Here's how the part is built. I have some questions about the finished solid (model axes, mm). A direction names the side the tool comes from. Give positions to 0.01 mm unless a question says otherwise; leave off trailing zeros. Loops run counter-clockwise (first coordinate to the right, second up) from the corner with the lowest first, then second, coordinate; pieces in that order, holes last. Notation, with made-up numbers: (15, -12.5) - (27, -12.5) arc R17 cw to (27, -6.5) - close; hole circle Ø5 at (-0.5, 2.25). An arc over 180 degrees is marked (long way). Return JSON: item names as keys, results as strings. Group by question number.
(1) If we mould it in two halves opening along Z, with no side actions, what happens to faces 1 (the flat face through (-12.834, 1.252, 106.011)), 2 (the flat face through (-2, 7, 177.8)), 3 (the flat face through (0, 170.384, 90))? For each: released by +Z, released by -Z, zero draft, split by the parting line, or undercut.
(2) If we section it at C-C (x = 79): Please give me the cut outline in (y, z).
(3) If we section it at A-A (z = 155.5): Please give me the cut outline in (x, y), then the cut area to 3 significant figures.
(4) If we section it at D-D (z = 114.3): Please give me the cut outline in (x, y).
(5) For P1, Ø8, axis at x = 5.5, z = 50, coming from the -Y side; P2, Ø2, axis at x = -41.5, y = 158.5, coming from the +Z side, each with a flat end and sliding along its axis, tell me the tip position at first contact or that it passes through.
(6) I need wall thicknesses on probe 1 along Y at (x, z) = (81.5, 143); probe 2 along X at (y, z) = (19, 147.5); probe 3 along Y at (x, z) = (8, 111). Which ranges of each line are inside material? Lowest first, please. Write a range as [from, to].
(7) On a 3-axis mill with a long thin cutter (end or side, diameter ignored), from which of +Z, -Z, +X, -X, +Y, -Y can I reach the whole of each face in a straight line? I mean faces 4 (the flat face through (24, 0, 88)), 5 (the flat face through (0, 93, 6.35)), 6 (the flat face through (12.834, 181.009, 106.011)), 7 (the flat face through (-24, 182.262, 88)), 8 (the flat face through (12.252, 1.252, 72.563)). Say none if no direction works.
(8) If we section it at B-B (y = 132.5): Please give me the cut outline in (x, z), then the cut area to 3 significant figures.
```python
from build123d import *

# Parameters (mm, degrees)
F1_DEPTH  = 177.8
F2_W      = 209.4248831272
F2_H      = 156.0155125335
F3_DEPTH  = 171.45
F4_W      = 155.5528063327
F4_H      = 6.91875844
F5_DEPTH  = 228.601
F6_W      = 2.54
F6_H      = 2.54
F7_DEPTH  = 228.601
F8_W      = 2.54
F8_H      = 2.54
F9_DEPTH  = 228.601
F10_W     = 8.4731229424
F10_H     = 0.6152642891
F11_DEPTH = 5.08
F12_W     = 10.7019939303
F12_H     = 0.6152642891
F13_DEPTH = 5.08
F14_W     = 0.6152642891
F14_H     = 2.54
F15_DEPTH = 228.601
F18_DEPTH = 2.54
F20_DEPTH = 2.54


with BuildPart() as f1:
    # F0 (on Top) → F1 (new body)
    with BuildSketch(Plane.XY):
        Polygon((-114.3, 0), (0, 0), (114.3, 0), (114.3, 182.2615116835), (-114.3, 182.2615116835), align=None)
    extrude(amount=F1_DEPTH)

    # F2 (on face) → F3 (cut)
    with BuildSketch(Plane.XY.offset(177.8)):
        with Locations((1.1144354939, 92.3765613697)):
            Rectangle(F2_W, F2_H)
    extrude(amount=-F3_DEPTH, mode=Mode.SUBTRACT)

    # F4 (on face) → F5 (cut, through all)
    with BuildSketch(Plane.YZ.offset(114.3)):
        with Locations((92.7604725584, 174.34062078)):
            Rectangle(F4_W, F4_H)
    extrude(amount=-F5_DEPTH, mode=Mode.SUBTRACT)

    # F6 (on face) → F7 (cut, through all)
    with BuildSketch(Plane.YZ.offset(114.3)):
        with Locations((171.8068757248, 172.15124156)):
            Rectangle(F6_W, F6_H)
    extrude(amount=-F7_DEPTH, mode=Mode.SUBTRACT)

    # F8 (on face) → F9 (cut, through all)
    with BuildSketch(Plane.YZ.offset(114.3)):
        with Locations((13.7140693921, 172.15124156)):
            Rectangle(F8_W, F8_H)
    extrude(amount=-F9_DEPTH, mode=Mode.SUBTRACT)

    # F10 (on face) → F11 (cut)
    with BuildSketch(Plane.XY.offset(177.8)):
        with Locations((110.0634385288, 14.6764372475)):
            Rectangle(F10_W, F10_H)
    extrude(amount=-F11_DEPTH, mode=Mode.SUBTRACT)

    # F12 (on face) → F13 (cut)
    with BuildSketch(Plane.XY.offset(177.8)):
        with Locations((-108.9490030348, 14.6764372475)):
            Rectangle(F12_W, F12_H)
    extrude(amount=-F13_DEPTH, mode=Mode.SUBTRACT)

    # F14 (on face) → F15 (cut, through all)
    with BuildSketch(Plane.YZ.offset(114.3)):
        with Locations((12.1364372475, 172.15124156)):
            Rectangle(F14_W, F14_H)
    extrude(amount=-F15_DEPTH, mode=Mode.SUBTRACT)

    # F17 (on face) → F18 (cut)
    with BuildSketch(Plane.XZ):
        with BuildLine():
            ThreePointArc((-0.6215579752, 38.1), (-0.3107789876, 38.0980988196), (0, 38.1))
            Line((0, 38.1), (-0.6215579752, 38.1))
        make_face()
        with BuildLine():
            Line((-0.6215579752, 38.1), (0, 38.1))
            ThreePointArc((0, 38.1), (15.1778442025, 43.3664673926), (24.1602391289, 56.6863478281))
            Line((24.1602391289, 56.6863478281), (0.0064452881, 88.8914062825))
            ThreePointArc((0.0064452881, 88.8914062825), (-0.8577674698, 88.8623323611), (-1.722469087, 88.8626440783))
            ThreePointArc((-1.722469087, 88.8626440783), (-25.7067084526, 62.9492276466), (-0.6215579752, 38.1))
        make_face()
        with BuildLine():
            ThreePointArc((-0.227703523, 88.9017653333), (-0.9753742254, 88.8932057202), (-1.722469087, 88.8626440783))
            ThreePointArc((-1.722469087, 88.8626440783), (-0.8577674698, 88.8623323611), (0.0064452881, 88.8914062825))
            Line((0.0064452881, 88.8914062825), (0, 88.9))
            ThreePointArc((0, 88.9), (-0.1138537398, 88.9006274972), (-0.227703523, 88.9017653333))
        make_face()
        with BuildLine():
            Line((0, 88.9), (0.0064452881, 88.8914062825))
            ThreePointArc((0.0064452881, 88.8914062825), (0.0862911744, 88.8955776847), (0.1661235568, 88.9))
            ThreePointArc((0.1661235568, 88.9), (0.0830617784, 88.8998641882), (0, 88.9))
        make_face()
        with BuildLine():
            ThreePointArc((0, 88.9), (-0.1138497834, 88.9011378184), (-0.227703523, 88.9017653333))
            ThreePointArc((-0.227703523, 88.9017653333), (-0.1138537398, 88.9006274972), (0, 88.9))
        make_face()
        with BuildLine():
            Line((-25.3127280516, 122.6503040688), (0, 88.9))
            ThreePointArc((0, 88.9), (0.0830617784, 88.8998641882), (0.1661235568, 88.9))
            ThreePointArc((0.1661235568, 88.9), (24.1602391289, 114.3), (0.1661235568, 139.7))
            Line((0.1661235568, 139.7), (0, 139.7))
            Line((0, 139.7), (-2.7280201219, 139.7))
            ThreePointArc((-2.7280201219, 139.7), (-16.6095490882, 134.6048766126), (-25.3127280516, 122.6503040688))
        make_face()
        with BuildLine():
            Line((0, 139.7), (0.1661235568, 139.7))
            ThreePointArc((0.1661235568, 139.7), (0.0830617784, 139.7001358118), (0, 139.7))
        make_face()
        with BuildLine():
            ThreePointArc((0, 139.7), (0.0830617784, 139.7001358118), (0.1661235568, 139.7))
            ThreePointArc((0.1661235568, 139.7), (-1.2809482826, 139.7411874115), (-2.7280201219, 139.7))
            Line((-2.7280201219, 139.7), (0, 139.7))
        make_face()
    extrude(amount=-F18_DEPTH, mode=Mode.SUBTRACT)

    # F19 (on face) → F20 (cut)
    with BuildSketch(Plane(origin=(0, 182.2615116835, 0), x_dir=(-1, 0, 0), z_dir=(0, 1, 0))):
        with BuildLine():
            ThreePointArc((-0.6215579752, 38.1), (-0.3107789876, 38.0980988196), (0, 38.1))
            Line((0, 38.1), (-0.6215579752, 38.1))
        make_face()
        with BuildLine():
            Line((-0.6215579752, 38.1), (0, 38.1))
            ThreePointArc((0, 38.1), (15.1778442025, 43.3664673926), (24.1602391289, 56.6863478281))
            Line((24.1602391289, 56.6863478281), (0.0064452881, 88.8914062825))
            ThreePointArc((0.0064452881, 88.8914062825), (-0.8577674698, 88.8623323611), (-1.722469087, 88.8626440783))
            ThreePointArc((-1.722469087, 88.8626440783), (-25.7067084526, 62.9492276466), (-0.6215579752, 38.1))
        make_face()
        with BuildLine():
            ThreePointArc((-0.227703523, 88.9017653333), (-0.9753742254, 88.8932057202), (-1.722469087, 88.8626440783))
            ThreePointArc((-1.722469087, 88.8626440783), (-0.8577674698, 88.8623323611), (0.0064452881, 88.8914062825))
            Line((0.0064452881, 88.8914062825), (0, 88.9))
            ThreePointArc((0, 88.9), (-0.1138537398, 88.9006274972), (-0.227703523, 88.9017653333))
        make_face()
        with BuildLine():
            Line((0, 88.9), (0.0064452881, 88.8914062825))
            ThreePointArc((0.0064452881, 88.8914062825), (0.0862911744, 88.8955776847), (0.1661235568, 88.9))
            ThreePointArc((0.1661235568, 88.9), (0.0830617784, 88.8998641882), (0, 88.9))
        make_face()
        with BuildLine():
            ThreePointArc((0, 88.9), (-0.1138497834, 88.9011378184), (-0.227703523, 88.9017653333))
            ThreePointArc((-0.227703523, 88.9017653333), (-0.1138537398, 88.9006274972), (0, 88.9))
        make_face()
        with BuildLine():
            Line((-25.3127280516, 122.6503040688), (0, 88.9))
            ThreePointArc((0, 88.9), (0.0830617784, 88.8998641882), (0.1661235568, 88.9))
            ThreePointArc((0.1661235568, 88.9), (24.1602391289, 114.3), (0.1661235568, 139.7))
            Line((0.1661235568, 139.7), (0, 139.7))
            Line((0, 139.7), (-2.7280201219, 139.7))
            ThreePointArc((-2.7280201219, 139.7), (-16.6095490882, 134.6048766126), (-25.3127280516, 122.6503040688))
        make_face()
        with BuildLine():
            Line((0, 139.7), (0.1661235568, 139.7))
            ThreePointArc((0.1661235568, 139.7), (0.0830617784, 139.7001358118), (0, 139.7))
        make_face()
        with BuildLine():
            ThreePointArc((0, 139.7), (0.0830617784, 139.7001358118), (0.1661235568, 139.7))
            ThreePointArc((0.1661235568, 139.7), (-1.2809482826, 139.7411874115), (-2.7280201219, 139.7))
            Line((-2.7280201219, 139.7), (0, 139.7))
        make_face()
    extrude(amount=-F20_DEPTH, mode=Mode.SUBTRACT)


solid = f1.part
```
Values:
{
 "1": {"face 1": "undercut", "face 2": "released by +Z", "face 3": "zero draft"},
 "2": {"outline": "(0, 0) - (182.26, 0) - (182.26, 177.8) - (170.54, 177.8) - (170.54, 173.42) - (173.08, 173.42) - (173.08, 170.88) - (170.38, 170.88) - (170.38, 6.35) - (14.37, 6.35) - (14.37, 170.88) - (11.83, 170.88) - (11.83, 173.42) - (14.37, 173.42) - (14.37, 177.8) - (0, 177.8) - close"},
 "3": {"outline": "(-114.3, 0) - (114.3, 0) - (114.3, 182.26) - (-114.3, 182.26) - close; hole (-103.6, 14.37) - (105.83, 14.37) - (105.83, 170.38) - (-103.6, 170.38) - close", "area": "8,990 mm2"},
 "4": {"outline": "(-114.3, 0) - (-19.05, 0) - (-19.05, 2.54) - (24.16, 2.54) - (24.16, 0) - (114.3, 0) - (114.3, 182.26) - (19.05, 182.26) - (19.05, 179.72) - (-24.16, 179.72) - (-24.16, 182.26) - (-114.3, 182.26) - close; hole (-103.6, 14.37) - (105.83, 14.37) - (105.83, 170.38) - (-103.6, 170.38) - close"},
 "5": {"P1": "y = 2.54", "P2": "z = 6.35"},
 "6": {"probe 1": "[0, 14.37], [170.38, 182.26]", "probe 2": "[-114.3, -103.6], [105.83, 114.3]", "probe 3": "[2.54, 14.37], [170.38, 179.72]"},
 "7": {"face 4": "+Z, -Z, +X, -X, -Y", "face 5": "+Z", "face 6": "+Y", "face 7": "+Z, -Z, +X, -X, +Y", "face 8": "-Y"},
 "8": {"outline": "(-114.3, 0) - (114.3, 0) - (114.3, 170.88) - (105.83, 170.88) - (105.83, 6.35) - (-103.6, 6.35) - (-103.6, 170.88) - (-114.3, 170.88) - close", "area": "4,610 mm2"}
}
